Source: CAD feature listing. Evaluate the final solid. Frame: model axes, mm. A direction names the side the tool comes from. Round coordinates to 2 decimals unless told otherwise and drop trailing zeros. Loops run counter-clockwise (first coordinate to the right, second up) from the corner with the lowest first, then second, coordinate; pieces in that order, holes last. Notation, with made-up numbers: (25.5, -40) - (78.5, -40) arc R36 ccw to (78.5, -4) - close; hole circle Ø3 at (1.25, -6). An arc over 180 degrees is marked (long way). One line per question, with ' | ' between items.
from build123d import *

# Parameters (mm, degrees)
F0_W      = 203
F0_H      = 86.0950331151
F1_DEPTH  = 50
F2_W      = 17.5
F2_H      = 45
F3_DEPTH  = 86.0960331151
F4_W      = 17.5
F4_H      = 45
F5_DEPTH  = 86.0960331151
F6_W      = 160
F6_H      = 46
F7_DEPTH  = 86.0960331151
F8_R      = 2
F9_W      = 78.5769208074
F9_H      = 46.412901438
F10_DEPTH = 25
F11_R     = 5


with BuildPart() as f1:
    # F0 (on Top) → F1 (new body)
    with BuildSketch(Plane.XY):
        with Locations((-0.5769208074, -2.0192312077)):
            Rectangle(F0_W, F0_H)
    extrude(amount=F1_DEPTH)

    # F2 (on face) → F3 (cut, through all)
    with BuildSketch(Plane.XZ.offset(45.0667477652)):
        with Locations((-93.3269208074, 22.5)):
            Rectangle(F2_W, F2_H)
    extrude(amount=-F3_DEPTH, mode=Mode.SUBTRACT)

    # F4 (on face) → F5 (cut, through all)
    with BuildSketch(Plane.XZ.offset(45.0667477652)):
        with Locations((92.1730791926, 22.5)):
            Rectangle(F4_W, F4_H)
    extrude(amount=-F5_DEPTH, mode=Mode.SUBTRACT)

    # F6 (on face) → F7 (cut, through all)
    with BuildSketch(Plane.XZ.offset(45.0667477652)):
        with Locations((-0.5769208074, 27)):
            Rectangle(F6_W, F6_H)
    extrude(amount=-F7_DEPTH, mode=Mode.SUBTRACT)

    # F8
    f8_edges = [f1.edges().sort_by_distance(p)[0] for p in [
        (79.423079, -2.019231, 50),
        (-80.576921, -2.019231, 50),
        (-84.576921, -2.019231, 45),
        (83.423079, -2.019231, 45),
        (79.423079, -2.019231, 4),
        (-80.576921, -2.019231, 4),
        (100.923079, -2.019231, 50),
        (-102.076921, -2.019231, 50),
    ]]
    fillet(f8_edges, radius=F8_R)

    # F9 (on face) → F10 (cut)
    with BuildSketch(Plane.XY.offset(4)):
        with Locations((-39.2884604037, 17.8218346309)):
            Rectangle(F9_W, F9_H)
    extrude(amount=-F10_DEPTH, mode=Mode.SUBTRACT)

    # F11
    f11_edges = [f1.edges().sort_by_distance(p)[0] for p in [
        (0, -5.384616, 2),
        (-78.576921, -5.384616, 2),
    ]]
    fillet(f11_edges, radius=F11_R)


solid = f1.part
1. Section query C-C, the plane y = -13. Return loops of the section in (x, z), plus the area to 4 significant figures.
Worked out:
outline: (-102.08, 45) - (-86.58, 45) arc R2 cw to (-84.58, 43) - (-84.58, 0) - (83.42, 0) - (83.42, 43) arc R2 cw to (85.42, 45) - (100.92, 45) - (100.92, 48) arc R2 ccw to (98.92, 50) - (81.42, 50) arc R2 ccw to (79.42, 48) - (79.42, 6) arc R2 cw to (77.42, 4) - (-78.58, 4) arc R2 cw to (-80.58, 6) - (-80.58, 48) arc R2 ccw to (-82.58, 50) - (-100.08, 50) arc R2 ccw to (-102.08, 48) - close | area: 1,215 mm2
2. Contact query for flat-ended pins moving along their axis: P1, Ø3, axis at y = 26, z = 1.5, coming from the +X side; P2, Ø1, axis at x = 46.5, y = 9, coming from the +Z side; P3, Ø8, axis at x = 96.5, y = 14, coming from the -Z side. Output: stop coordinate, or through.
Worked out:
P1: stops at x = 83.42 | P2: stops at z = 4 | P3: stops at z = 45
3. Section query D-D, the plane x = -66.5. Return loops of the section in (y, z), plus the area to 3 significant figures.
Worked out:
outline: (-45.07, 0) - (-5.38, 0) - (-5.38, 4) - (-45.07, 4) - close | area: 159 mm2
4. Access query for faces 4 (the flat face through (-80.577, -3, 27)), 5 (the flat face through (-78.577, 20, 2)), 6 (the flat face through (93, -3, 45)), 7 (the flat face through (-84.577, -3, 21)), 8 (the flat face through (-9, -45.067, 3)). Directions: +Z, -Z, +X, -X, +Y, -Y. A direction counts if a zero-diameter tool reaches every point of the face in a straight line with its end or side. Return the directions, or none.
Worked out:
face 4: +Z, +Y, -Y | face 5: +Z, -Z, +Y | face 6: -Z, +X, +Y, -Y | face 7: -Z, -X, +Y, -Y | face 8: +Z, -Z, +X, -X, -Y
5. Section query A-A, the plane y = 4.5. Return loops of the section in (x, z), plus the area to 3 significant figures.
Worked out:
outline: (-102.08, 45) - (-86.58, 45) arc R2 cw to (-84.58, 43) - (-84.58, 0) - (-78.58, 0) - (-78.58, 4) arc R2 cw to (-80.58, 6) - (-80.58, 48) arc R2 ccw to (-82.58, 50) - (-100.08, 50) arc R2 ccw to (-102.08, 48) - close; (0, 0) - (83.42, 0) - (83.42, 43) arc R2 cw to (85.42, 45) - (100.92, 45) - (100.92, 48) arc R2 ccw to (98.92, 50) - (81.42, 50) arc R2 ccw to (79.42, 48) - (79.42, 6) arc R2 cw to (77.42, 4) - (0, 4) - close | area: 901 mm2
6. Material intervals for probe 1 along X at (y, z) = (13, 16); probe 2 along Z at (x, y) = (33, 12.5), sorted ascending.
Worked out:
probe 1: x = -84.58 to -80.58, 79.42 to 83.42 | probe 2: z = 0 to 4
7. Section query B-B, the plane z = 37. Return loops of the section in (x, y).
Worked out:
outline: (-84.58, -45.07) - (-80.58, -45.07) - (-80.58, 41.03) - (-84.58, 41.03) - close; (79.42, -45.07) - (83.42, -45.07) - (83.42, 41.03) - (79.42, 41.03) - close
8. Mould query, pull axis X, two halves, no side actions, for faces 1 (the flat face through (0, 20, 2)), 2 (the flat face through (83.423, -3, 21)), 3 (the flat face through (-94, -3, 45)). Classes: released by +X, released by -X, zero draft, split by the parting line, or undercut.
Worked out:
face 1: undercut | face 2: released by +X | face 3: zero draft
